Build history of the part. All positions in model axes, mm. A direction names the side the tool comes from. Round coordinates to 2 decimals unless told otherwise and drop trailing zeros. Write each loop counter-clockwise with the first axis right and the second up, starting at its lowest first coordinate (ties: lowest second). Pieces come first, ordered by that corner, then holes. Notation, with made-up numbers: M 87,23.5 L 107,23.5 A35 ccw 107,60.5 Z; hole C 5.5,-33.75 d4. An arc over 180 degrees is marked long. Write item = value, one per line. Start each with the question number.
Q1. Band-saw the part on C-C on x = -19. Write the cut outline in (y, z), plus the area to 3 significant figures.
Q2. Band-saw the part on B-B on y = -9. Write the cut outline in (x, z), plus the area to 3 significant figures.
Q3. Pull direction Z, two halves, no side cores. Call faces 1 (the flat face through (27, 2.9, 1)), 2 (the cylindrical face through (16.32, -11.85, 1.87)), 3 (the flat face through (34.8, 0.1, 0.5)), 4 (the cylindrical face through (31.792, -1.181, -1.232)): released by +Z, released by -Z, zero draft, split by the parting line, or undercut.
Q4. Band-saw the part on A-A on z = 7.5. Write the cut outline in (x, y), plus the area to 3 significant figures.
Q5. Tool access for faces 5 (the flat face through (36, -4.05, -1)), 6 (the cylindrical face through (4.07, -3.9, 1.9)), 7 (the flat face through (29.5, -14, 7)), 8 (the flat face through (34.5, 2, -3)), 9 (the flat face through (-10, 4, 3.5)): list every direction of +Z, -Z, +X, -X, +Y, -Y with a clear straight run to the whole face (end or side of a thin tool).
Q6. Band-saw the part on D-D on y = 6. Write the cut outline in (x, z), plus the area to 3 significant figures.
Q7. Probe L1, parallel to Y at x = -1.5, z = 1.3; L2, parallel to Y at x = 36.25, z = 1.8; L3, parallel to Z at x = 1, y = 8.5. List the from-to ranges inside material, lowest first.
Q8. Drop flat-ended pins along their axis: P1, Ø10, axis at x = -3.5, y = -3, coming from the +Z side; P2, Ø1, axis at x = -9.5, z = 4.5, coming from the +Y side; P3, Ø10, axis at x = 21.5, y = -3.5, coming from the +Z side; P4, Ø4, axis at y = -10, z = 1.5, coming from the +X side. Give the stop position or say it passes through.
Autodesk Inventor part; units mm, degrees
ref_plane "YZ Plane" through (0, 0, 0) normal (1, 0, 0) x (0, 1, 0)
ref_plane "XZ Plane" through (0, 0, 0) normal (0, 1, 0) x (-1, 0, 0)
ref_plane "XY Plane" through (0, 0, 0) normal (0, 0, 1) x (1, 0, 0)
sketch "Sketch1" plane through (0, 0, 0) normal (0, 0, 1) x (1, 0, 0)
  arc A0 (-20, 13.65) -> (-13.5, 20.15) centre (-20, 20.15) ccw
  circle A1 centre (-20, 20.15) radius 4.5
  arc A2 (-20, 13.65) -> (-22.5, 11.15) centre (-20, 11.15) ccw
  line L0 (-22.5, 11.15) -> (-22.5, -15.45)
  circle A3 centre (-19, -1.2) radius 1.5
  line L1 (-22.5, -15.45) -> (-15, -15.45)
  line L2 (34.5, -7.1) -> (34.5, 2.9)
  line L3 (34.5, 2.9) -> (32, 2.9)
  arc A4 (3.45, 17.7) -> (-1.5, 22.65) centre (-1.5, 17.7) ccw
  circle A5 centre (-1.5, 17.7) radius 1.5
  arc A6 (-11, 22.65) -> (-13.5, 20.15) centre (-11, 20.15) ccw
  line L4 (-11, 22.65) -> (-1.5, 22.65)
  arc A7 (3.45, 5.4) -> (5.95, 2.9) centre (5.95, 5.4) ccw
  line L5 (3.45, 5.4) -> (3.45, 17.7)
  circle A8 centre (23.5, 7.6) radius 2.7
  line L6 (-15, -15.45) -> (32, -15.45)
  line L7 (32, 20.05) -> (32, 2.9) construction
  line L8 (32, 2.9) -> (5.95, 2.9)
  line L9 (32, -15.45) -> (32, -7.1)
  line L10 (32, -7.1) -> (34.5, -7.1)
  point P0 (0, 0)
  point P1 (-32, -15.45)
  dimension "d0" = 90
  dimension "d1" = 90
  dimension "d2" = 2
  dimension "d3" = 3.5
  dimension "d5" = 90
  dimension "d6" = 90
  dimension "d7" = 4.7
  dimension "d51" = 2.5
  dimension "d52" = 10
extrude "Extrusion1" add sketch "Sketch1" along normal blind 3.5 contours A0 A6 L4 A4 L5 A7 L8 L3 L2 L10 L9 L6 L1 L0 A2
sketch "Sketch2" plane through (0, 0, 3.5) normal (0, 0, 1) x (1, 0, 0)
  line L0 (29.5, 12.55) -> (29.5, -12.45)
  line L1 (29.5, -12.45) -> (3.5, -12.45)
  line L2 (29.5, 12.55) -> (3.5, 12.55)
  line L3 (3.5, 12.55) -> (3.5, -12.45)
  point P0 (0, 0)
  point P1 (6.5, -20.5)
  point P2 (26.5, -20.5)
  point P3 (32, -15.45)
  dimension "d14" = 3
  dimension "d15" = 3
  dimension "d16" = 25
  dimension "d53" = 2.5
  dimension "d54" = 3
extrude "Extrusion2" cut sketch "Sketch2" against normal blind 2.2
fillet "Fillet1" radius 2 3 edges at (16.5, -12.45, 1.3) (3.5, -3.7737, 1.3) (29.5, -4.775, 1.3)
sketch "Sketch3" plane through (-15, -15.45, 0) normal (0, -1, 0) x (1, 0, 0)
  circle A0 centre (31.5, 10.5) radius 4.3 construction
  line L0 (39.5, 4.5) -> (23.5, 4.5)
  arc A1 (39.5, 4.5) -> (39.5, 16.5) centre (31.5, 10.5) ccw
  line L1 (23.5, 16.5) -> (39.5, 16.5)
  arc A2 (23.5, 16.5) -> (23.5, 4.5) centre (31.5, 10.5) ccw
  line L2 (39.6976, 16.9) -> (23.3024, 16.9) construction
  line L3 (39.6976, 4.1) -> (23.3024, 4.1)
  arc A3 (39.6976, 4.1) -> (41.888, 10) centre (31.5, 10.5) ccw
  arc A4 (23.3024, 16.9) -> (21.1, 10.5) centre (31.5, 10.5) ccw construction
  line L4 (41.9, 3.5) -> (21.1, 3.5)
  line L5 (21.1, 3.5) -> (21.1, 10.5) construction
  line L6 (41.9, 3.5) -> (41.9, 10.5) construction
  arc A5 (41.9, 10.5) -> (39.6976, 16.9) centre (31.5, 10.5) ccw construction
  arc A6 (21.1, 10.5) -> (21.112, 10) centre (31.5, 10.5) ccw construction
  line L7 (21.1, 10.5) -> (18.5, 10.5) construction
  line L8 (18.5, 10.5) -> (18.5, 10) construction
  line L9 (18.5, 3.5) -> (21.1, 3.5)
  line L10 (41.9, 10.5) -> (44.5, 10.5) construction
  line L11 (44.5, 10.5) -> (44.5, 10) construction
  line L12 (44.5, 3.5) -> (41.9, 3.5)
  line L13 (21.112, 10) -> (18.5, 10)
  line L14 (18.5, 10) -> (18.5, 3.5)
  arc A7 (21.112, 10) -> (23.3024, 4.1) centre (31.5, 10.5) ccw
  line L15 (41.888, 10) -> (44.5, 10)
  arc A8 (41.888, 10) -> (41.9, 10.5) centre (31.5, 10.5) ccw construction
  line L16 (44.5, 10) -> (44.5, 3.5)
  point P0 (15, 0)
  point P1 (19.806, 10)
  point P2 (43.194, 10)
  dimension "d22" = 0.4
  dimension "d23" = 0.4
  dimension "d55" = 6.5
extrude "Extrusion3" add sketch "Sketch3" against normal blind 3 contours A3 L15 L16 L12 L4 L9 L14 L13 A7 L3
sketch "Sketch4" plane through (0, 0, 0) normal (0, 0, -1) x (-1, 0, 0)
  line L0 (-32, -15.45) -> (-32, 20.05)
  line L1 (-34.5, -7.1) -> (-34.5, 2.9)
  line L2 (22.5, 11.15) -> (22.5, -15.45)
  arc A0 (22.5, 11.15) -> (20, 13.65) centre (20, 11.15) ccw
  arc A1 (13.5, 20.15) -> (20, 13.65) centre (20, 20.15) ccw
  arc A2 (13.5, 20.15) -> (11, 22.65) centre (11, 20.15) ccw
  line L3 (1.5, 22.65) -> (11, 22.65)
  arc A3 (1.5, 22.65) -> (-3.45, 17.7) centre (1.5, 17.7) ccw
  line L4 (-3.45, 5.4) -> (-3.45, 17.7)
  arc A4 (-5.95, 2.9) -> (-3.45, 5.4) centre (-5.95, 5.4) ccw
  line L5 (-34.5, 2.9) -> (-5.95, 2.9)
  line L6 (-34.5, -7.1) -> (-34.5, 2.9)
  line L7 (-32, -7.1) -> (-34.5, -7.1)
  line L8 (-32, -15.45) -> (-32, -7.1)
  line L9 (22.5, -15.45) -> (-32, -15.45)
  circle A5 centre (19, -1.2) radius 1.5
  circle A6 centre (1.5, 17.7) radius 1.5
  line L10 (-32, -7.1) -> (-34.5, -7.1)
  point P0 (0, 0)
  point P1 (-32, 2.9)
extrude "Extrusion4" add sketch "Sketch4" along normal blind 4.05 contours L7 L1 L5 L0
sketch "Sketch5" plane through (32, -15.45, 0) normal (-1, 0, 0) x (0, 0, 1)
  line L0 (-4.05, 18.35) -> (-2.55, 18.35)
  line L1 (-2.55, 18.35) -> (-2.55, 8.35)
  line L2 (-2.55, 8.35) -> (-4.05, 8.35)
  line L3 (-4.05, 8.35) -> (-4.05, 18.35)
  point P0 (0, 15.45)
  dimension "d57" = 1.5
extrude "Extrusion5" add sketch "Sketch5" along normal blind 5
sketch "Sketch8" plane through (0, 0, 3.5) normal (0, 0, 1) x (1, 0, 0)
  circle A0 centre (36.25, -1.2) radius 1.7
  arc A1 (36.25, -5.3) -> (36.25, 2.9) centre (36.25, -1.2) ccw
  line L0 (36.25, 2.9) -> (34.5, 2.9)
  line L1 (36.25, -5.3) -> (34.5, -5.3)
  arc A2 (34.5, 2.9) -> (34.5, -5.3) centre (36.25, -1.2) ccw
  point P0 (0, 0)
  dimension "d35" = 3.4
  dimension "d36" = 2.4
  dimension "d37" = 1.75
extrude "Extrusion7" add sketch "Sketch8" against normal blind 6
sketch "Sketch9" plane through (0, 0, -2.5) normal (0, 0, -1) x (-1, 0, 0)
  line L0 (-34.6046, -4.05) -> (-37.8954, -4.05)
  line L1 (-37.8954, -4.05) -> (-39.5409, -1.2)
  line L2 (-39.5409, -1.2) -> (-37.8954, 1.65)
  line L3 (-37.8954, 1.65) -> (-34.6046, 1.65)
  line L4 (-34.6046, 1.65) -> (-32.9591, -1.2)
  line L5 (-32.9591, -1.2) -> (-34.6046, -4.05)
  circle A0 centre (-36.25, -1.2) radius 1.7
  point P0 (0, 0)
  point P1 (-36.25, -1.2)
  point P2 (-34.5, -2.718)
  point P3 (-34.5, -0.482)
  point P4 (-34.5, -0.4601)
  point P5 (-34.5, -1.9399)
  dimension "d42" = 5.7
extrude "Extrusion9" cut sketch "Sketch9" along normal blind 6 and the other way blind 3 contours L0 L1 L2 L3 L4 L5 | A0
sketch "Sketch10" plane through (5.95, 2.9, 1.3) normal (0, 1, 0) x (1, 0, 0)
  line L0 (26.05, 3.8) -> (26.05, 1.3)
  line L1 (26.2, 1.3) -> (26.2, 3.8)
  line L2 (26.2, 3.8) -> (26.05, 3.8)
  line L3 (26.05, 1.3) -> (26.2, 1.3)
  point P0 (-5.95, 1.3)
  dimension "d47" = 0.15
extrude "Extrusion10" cut sketch "Sketch10" against normal blind 10
properties part number "BACKPLATE" material "PET Plastic"
Conclusion:
q1.outline = M -15.45,0 L -2.7,0 L -2.7,3.5 L -15.45,3.5 Z; M 0.3,0 L 13.73,0 L 13.73,3.5 L 0.3,3.5 Z
q1.area = 91.6 mm^2
q2.outline = M -22.5,0 L 32,0 L 32,3.5 L 29.5,3.5 L 29.5,3.3 A2 cw 27.5,1.3 L 5.5,1.3 A2 cw 3.5,3.3 L 3.5,3.5 L -22.5,3.5 Z
q2.area = 135 mm^2
q3.face_1 = zero draft
q3.face_2 = released by +Z
q3.face_3 = released by -Z
q3.face_4 = undercut
q4.outline = M 3.5,-15.45 L 6.54,-15.45 L 6.54,-12.45 L 3.5,-12.45 Z; M 26.46,-15.45 L 29.5,-15.45 L 29.5,-12.45 L 26.46,-12.45 Z
q4.area = 18.3 mm^2
q5.face_5 = -Z
q5.face_6 = +Z, +Y
q5.face_7 = +Z, +X, +Y, -Y
q5.face_8 = -Z, +X, +Y, -Y
q5.face_9 = +Z, -X, +Y, -Y
q6.outline = M -22.5,0 L 3.45,0 L 3.45,3.5 L -22.5,3.5 Z
q6.area = 90.8 mm^2
q7.L1 = -15.45 to 16.2, 19.2 to 22.65
q7.L2 = -5.3 to -2.9, 0.5 to 2.9
q7.L3 = 0 to 3.5
q8.P1 = 3.5
q8.P2 = through
q8.P3 = 1.3
q8.P4 = 32
